Input: part model. Units: mm. Frame: model coordinates. Face numbers are marked on the shaded views. A direction names the side the tool comes from. Coordinates: 2 decimals unless noted, no trailing zeros. Loops run counter-clockwise (first coordinate to the right, second up) from the corner with the lowest first, then second, coordinate; pieces in that order, holes last. Notation, with made-up numbers: M 42,68 L 80,68 A17 cw 80,80 Z; hole C -21.75,5.5 d11. An arc over 180 degrees is marked long. Use a Markdown table: item, result. Add a question column.
1. Pin query (flat end, axial travel): pin 1 (4 mm diameter, centred on x = 22.44, z = 8, fed in from -Y); pin 2 (0.8 mm diameter, centred on x = 0, z = 1.5, fed in from -Y); pin 3 (4 mm diameter, centred on x = 22.44, z = 8, fed in from +Y). Return the tip coordinate at first contact, or that it passes through.
2. Draft query along X for the marked faces 3, 4 and 5. Return one class per face: +X half, -X half, draft (parallel to the pull), parting line (faces both ways), or undercut.
3. Line query: L1, parallel to Y at x = 0, z = 10; L2, parallel to Z at x = 35.5, y = 4.5; L3, parallel to Z at x = 22, y = -2. Output: solid intervals per line, ascending. Write a range as [from, to].
4. Set-up query: the marked faces 1 and 2. Return all of +Z, -Z, +X, -X, +Y, -Y with unobstructed straight access to the full face (end or side cutting, diameter ignored); none if empty.
5. Section C-C on y = 23.5. Output: boundary loops of the cut face in (x, z), then the cut area to 3 significant figures.
6. Section A-A on z = 8. Output: boundary loops of the cut face in (x, y), then the cut area to 3 significant figures.
7. Section B-B on y = -28. Output: boundary loops of the cut face in (x, z).
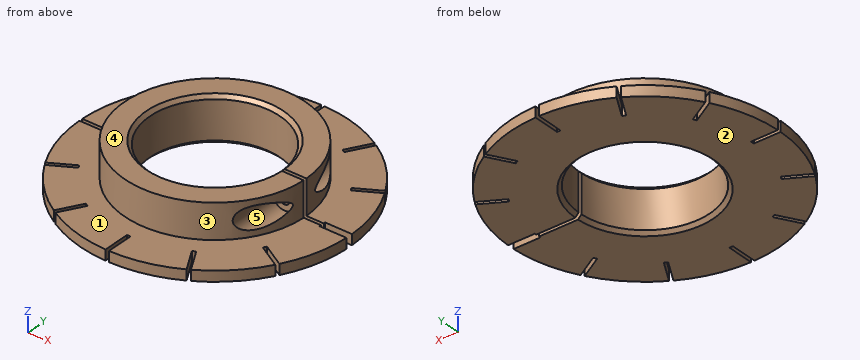
Autodesk Inventor part; units mm, degrees
ref_plane "Work Plane1" through (18.7433, 3, 13) normal (0, -1, 0) x (1, 0, 0)
ref_plane "YZ Plane" through (0, 0, 0) normal (1, 0, 0) x (0, 1, 0)
ref_plane "XZ Plane" through (0, 0, 0) normal (0, 1, 0) x (-1, 0, 0)
sketch "Sketch1" plane through (0, 0, 0) normal (0, 0, 1) x (1, 0, 0)
  circle A0 centre (0, 0) radius 38.75
  line L0 (-0.5, 39) -> (0.5, 39)
  line L1 (0.5, 39) -> (0.5, 31)
  line L2 (0.5, 31) -> (-0.5, 31)
  line L3 (-0.5, 31) -> (-0.5, 39)
  line L4 (-15.933, 26.5968) -> (-19.933, 33.525)
  line L5 (-19.067, 34.025) -> (-15.067, 27.0968)
  line L6 (-15.067, 27.0968) -> (-15.933, 26.5968)
  line L7 (-19.933, 33.525) -> (-19.067, 34.025)
  line L8 (-27.0968, 15.067) -> (-34.025, 19.067)
  line L9 (-33.525, 19.933) -> (-26.5968, 15.933)
  line L10 (-26.5968, 15.933) -> (-27.0968, 15.067)
  line L11 (-34.025, 19.067) -> (-33.525, 19.933)
  line L12 (-31, -0.5) -> (-39, -0.5)
  line L13 (-39, 0.5) -> (-31, 0.5)
  line L14 (-31, 0.5) -> (-31, -0.5)
  line L15 (-39, -0.5) -> (-39, 0.5)
  line L16 (-26.5968, -15.933) -> (-33.525, -19.933)
  line L17 (-34.025, -19.067) -> (-27.0968, -15.067)
  line L18 (-27.0968, -15.067) -> (-26.5968, -15.933)
  line L19 (-33.525, -19.933) -> (-34.025, -19.067)
  line L20 (-15.067, -27.0968) -> (-19.067, -34.025)
  line L21 (-19.933, -33.525) -> (-15.933, -26.5968)
  line L22 (-15.933, -26.5968) -> (-15.067, -27.0968)
  line L23 (-19.067, -34.025) -> (-19.933, -33.525)
  line L24 (0.5, -31) -> (0.5, -39)
  line L25 (-0.5, -39) -> (-0.5, -31)
  line L26 (-0.5, -31) -> (0.5, -31)
  line L27 (0.5, -39) -> (-0.5, -39)
  line L28 (15.933, -26.5968) -> (19.933, -33.525)
  line L29 (19.067, -34.025) -> (15.067, -27.0968)
  line L30 (15.067, -27.0968) -> (15.933, -26.5968)
  line L31 (19.933, -33.525) -> (19.067, -34.025)
  line L32 (27.0968, -15.067) -> (34.025, -19.067)
  line L33 (33.525, -19.933) -> (26.5968, -15.933)
  line L34 (26.5968, -15.933) -> (27.0968, -15.067)
  line L35 (34.025, -19.067) -> (33.525, -19.933)
  line L36 (31, 0.5) -> (39, 0.5)
  line L37 (39, -0.5) -> (31, -0.5)
  line L38 (31, -0.5) -> (31, 0.5)
  line L39 (39, 0.5) -> (39, -0.5)
  line L40 (26.5968, 15.933) -> (33.525, 19.933)
  line L41 (34.025, 19.067) -> (27.0968, 15.067)
  line L42 (27.0968, 15.067) -> (26.5968, 15.933)
  line L43 (33.525, 19.933) -> (34.025, 19.067)
  line L44 (15.067, 27.0968) -> (19.067, 34.025)
  line L45 (19.933, 33.525) -> (15.933, 26.5968)
  line L46 (15.933, 26.5968) -> (15.067, 27.0968)
  line L47 (19.067, 34.025) -> (19.933, 33.525)
  point P0 (0, 31)
  point P1 (-0.5, 38.7468)
  point P2 (0.5, 38.7468)
  point P3 (-15.5, 26.8468)
  point P4 (-26.8468, 15.5)
  point P5 (-31, 0)
  point P6 (-26.8468, -15.5)
  point P7 (-15.5, -26.8468)
  point P8 (0, -31)
  point P9 (15.5, -26.8468)
  point P10 (26.8468, -15.5)
  point P11 (31, 0)
  point P12 (26.8468, 15.5)
  point P13 (15.5, 26.8468)
  point P14 (-18.9404, 33.8057)
  point P15 (-19.8064, 33.3057)
  point P16 (-33.3057, 19.8064)
  point P17 (-33.8057, 18.9404)
  point P18 (-38.7468, 0.5)
  point P19 (-38.7468, -0.5)
  point P20 (-33.8057, -18.9404)
  point P21 (-33.3057, -19.8064)
  point P22 (-19.8064, -33.3057)
  point P23 (-18.9404, -33.8057)
  point P24 (-0.5, -38.7468)
  point P25 (0.5, -38.7468)
  point P26 (18.9404, -33.8057)
  point P27 (19.8064, -33.3057)
  point P28 (33.3057, -19.8064)
  point P29 (33.8057, -18.9404)
  point P30 (38.7468, -0.5)
  point P31 (38.7468, 0.5)
  point P32 (33.8057, 18.9404)
  point P33 (33.3057, 19.8064)
  point P34 (19.8064, 33.3057)
  point P35 (18.9404, 33.8057)
  dimension "d0" = 77.5
  dimension "d1" = 1
  dimension "d2" = 8
  dimension "d3" = 0.5
  dimension "d4" = 31
  dimension "d9" = 360
extrude "Extrusion1" add sketch "Sketch1" along normal blind 3 contours L36 L38 L37 A0 L32 L34 L33 L28 L30 L29 L24 L26 L25 L20 L22 L21 L16 L18 L17 L12 L14 L13 L8 L10 L9 L4 L6 L5 L3 L2 L1 L44 L46 L45 L40 L42 L41
sketch "Sketch2" plane through (0, 0, 3) normal (0, 0, 1) x (1, 0, 0)
  circle A0 centre (0, 0) radius 18.75
  circle A1 centre (0, 0) radius 26
  dimension "d11" = 37.5
  dimension "d12" = 52
extrude "Extrusion2" add sketch "Sketch2" along normal blind 10
sketch "Sketch3" plane through (0, 0, 3) normal (0, 0, 1) x (1, 0, 0)
  circle A0 centre (0, 0) radius 18.75
extrude "Extrusion3" cut sketch "Sketch3" against normal blind 10
sketch "Sketch4" plane through (0, 0, 13) normal (0, 0, 1) x (1, 0, 0)
  arc A0 (33.8057, -18.9404) -> (38.7468, -0.5) centre (0, 0) ccw
  line L0 (38.7468, -0.5) -> (17.4484, -0.5)
  line L1 (17.4484, -0.5) -> (17.4484, 0.5)
  line L2 (17.4484, 0.5) -> (38.7468, 0.5)
  line L3 (38.7468, 0.5) -> (38.7468, -0.5)
  line L4 (31, 1) -> (40.0251, 1)
  line L5 (40.0251, 1) -> (40.0251, -1)
  line L6 (40.0251, -1) -> (31, -1)
  line L7 (31, -1) -> (31, 1)
  point P0 (31, -0.5)
  point P1 (31, 0.5)
  dimension "d19" = 2
  dimension "d20" = 0.5
extrude "Extrusion4" cut sketch "Sketch4" against normal through all
sketch "Sketch5" plane through (18.7433, 0.5, 13) normal (0, -1, 0) x (1, 0, 0)
  circle A0 centre (3.7, -5) radius 1.6
  line L0 (14.5624, -10) -> (1.0631, -10)
  line L1 (-37.4933, 0) -> (0, 0)
  line L2 (0, 0) -> (0, -10)
  point P0 (-18.7433, -13)
  point P1 (0, -5)
  dimension "d21" = 3.2
  dimension "d22" = 5
  dimension "d23" = 3.7
extrude "Extrusion5" cut sketch "Sketch5" against normal blind 23.5
ref_plane "Work Plane1" through (18.7433, 3, 13) normal (0, -1, 0) x (1, 0, 0)
sketch "Sketch6" plane through (18.7433, 3, 13) normal (0, -1, 0) x (1, 0, 0)
  circle A0 centre (3.7, -5) radius 1.6
  circle A1 centre (3.7, -5) radius 3.25
  point P0 (-18.7433, -13)
  dimension "d27" = 6.5
extrude "Extrusion6" cut sketch "Sketch6" against normal blind 23.5
mirror "Mirror1" about plane through (0, 0, 0) normal (0, 1, 0) of "Extrusion6", "Extrusion5"
chamfer "Chamfer1" distance 1 angle 45 2 edges at (-18.75, 0, 13) (-18.75, 0, 0)
properties part number "disk_12_slot"
Answers below:
| question | item | result |
|---|---|---|
| 1 | pin 1 | stops at y = -3 |
| 1 | pin 2 | stops at y = -31 |
| 1 | pin 3 | stops at y = 3 |
| 2 | face 3 | parting line |
| 2 | face 4 | draft |
| 2 | face 5 | undercut |
| 3 | L1 | y = [-26, -18.75], [18.75, 26] |
| 3 | L2 | z = [0, 3] |
| 3 | L3 | z = [0, 6.46], [9.54, 13] |
| 4 | face 1 | +Z |
| 4 | face 2 | -Z, +X, -X, +Y, -Y |
| 5 | outline | M -30.81,0 L 30.81,0 L 30.81,3 L 11.12,3 L 11.12,13 L -11.12,13 L -11.12,3 L -30.81,3 Z |
| 5 | area | 407 mm² |
| 6 | outline | M 18.74,-0.5 A18.75 cw long 18.74,0.5 L 20.84,0.5 L 20.84,3 L 19.19,3 L 19.19,17.54 A26 ccw long 19.19,-17.54 L 19.19,-3 L 20.84,-3 L 20.84,-0.5 Z; M 24.04,-3 L 25.69,-3 L 25.69,-3.98 A26 ccw 26,-0.5 L 24.04,-0.5 Z; M 24.04,0.5 L 26,0.5 A26 ccw 25.69,3.98 L 25.69,3 L 24.04,3 Z |
| 6 | area | 873 mm² |
| 7 | outline | M -26.79,0 L -16.74,0 L -16.74,3 L -26.79,3 Z; M -15.59,0 L 15.59,0 L 15.59,3 L -15.59,3 Z; M 16.74,0 L 26.79,0 L 26.79,3 L 16.74,3 Z |
